The figure shows three views and two pictorial views of one solid part (mm, origin at its lowest corner). Answer the questions. Give positions to 0.01 mm unless a question says otherwise; leave off trailing zeros. Loops run counter-clockwise (first coordinate to the right, second up) from the corner with the lowest first, then second, coordinate; pieces in that order, holes last. Notation, with made-up numbers: (-16.5, -13) - (-1.5, -13) arc R20 cw to (-1.5, 3) - close; hole circle Ø2 at (27.25, -6). An arc over 180 degrees is marked (long way). One line per question, with ' | ' between items.
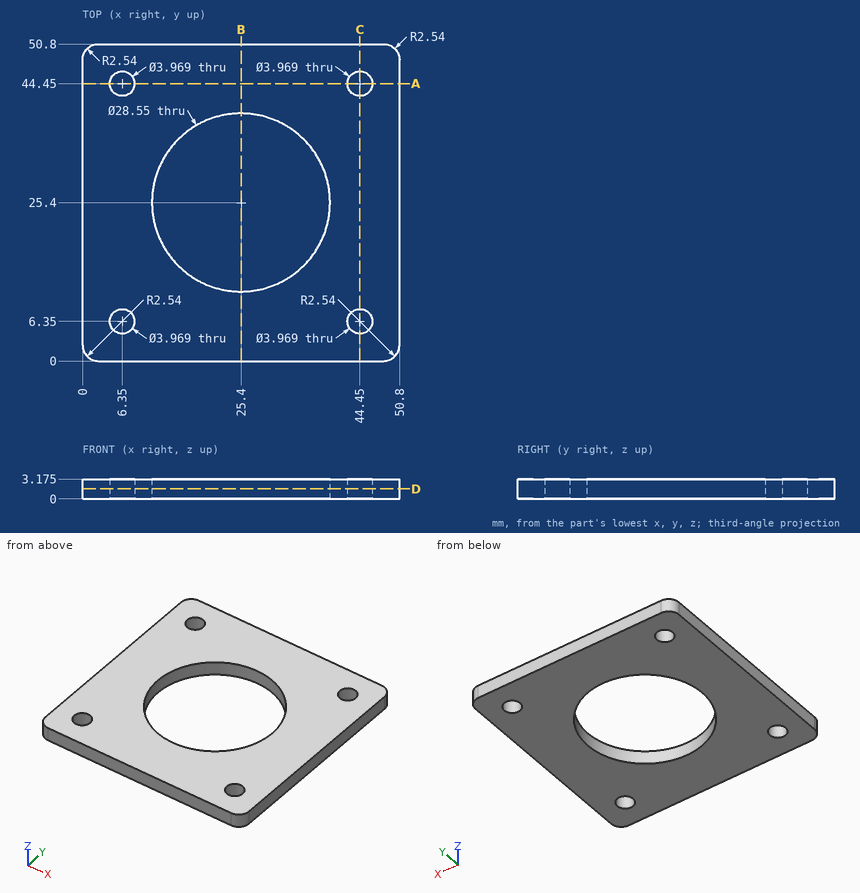
1. Find section D-D on z = 1.6. State how many separate pieces and enclosed holes the cut face has, then the cut area to 3 significant figures.
Evaluation:
separate pieces: 1 | enclosed holes: 5 | area: 1,890 mm2
2. A flat-ended cylindrical pin translates along its axis: pin 1 (2.5 mm diameter, centred on x = 6.35, y = 44.45, fed in from -Z). Find the tip coordinate at first contact, or state that the pin passes through.
Evaluation:
pin 1: through
3. Find section A-A on y = 44.45. Write down the section's boundary in (x, z) (1 decimal), then the cut area to 3 significant figures.
Evaluation:
outline: (0, 0) - (4.4, 0) - (4.4, 3.2) - (0, 3.2) - close; (8.3, 0) - (42.5, 0) - (42.5, 3.2) - (8.3, 3.2) - close; (46.4, 0) - (50.8, 0) - (50.8, 3.2) - (46.4, 3.2) - close | area: 136 mm2
4. Find section B-B on x = 25.4. Write down the section's boundary in (y, z) (1 decimal).
Evaluation:
outline: (0, 0) - (11.1, 0) - (11.1, 3.2) - (0, 3.2) - close; (39.7, 0) - (50.8, 0) - (50.8, 3.2) - (39.7, 3.2) - close
5. Consider L1, parallel to Y at x = 6.35, z = 2.5 (1 decimal); L2, parallel to Y at x = 25.4, z = 1.2 (1 decimal); L3, parallel to Y at x = 7, z = 2.65 (1 decimal). Determine where each line is inside the solid, lowest interval first.
Evaluation:
L1: 0 to 4.4, 8.3 to 42.5, 46.4 to 50.8 | L2: 0 to 11.1, 39.7 to 50.8 | L3: 0 to 4.5, 8.2 to 42.6, 46.3 to 50.8
